The listing builds one solid part. Answer for the finished solid, in the listing's coordinates (mm). A direction names the side the tool comes from. Coordinates: 2 decimals unless noted, no trailing zeros. Order: outer loops, then holes, each group sorted by start corner. A loop starts at its lowest first (then second) coordinate and runs counter-clockwise, first axis right, second up. Notation, with made-up numbers: (18.5, 21.5) -> (53.5, 21.5) arc R14 ccw to (53.5, 27.5) -> close; hole circle Ø2 at (25.25, 50). An arc over 180 degrees is marked (long way). Return JSON: item names as keys, results as strings.
```python
from build123d import *

# Parameters (mm, degrees)
BOSS_EXTRUDE1_DEPTH     = 130
CUT_EXTRUDE3_DEPTH      = 273.019096875
CUT_EXTRUDE3_DEPTH_BACK = 273.019096875
FILLET2_SIZE            = 10
CUT_EXTRUDE4_DEPTH      = 272.254010875
CUT_EXTRUDE4_DEPTH_BACK = 272.254010875
SKETCH8_R               = 1.5
SKETCH9_W               = 24.273397223
SKETCH9_H               = 9.918939499
BOSS_EXTRUDE5_DEPTH     = 129
FILLET5_SIZE            = 5


with BuildPart() as part:
    # Sketch1 → Boss-Extrude1 (new body)
    with BuildSketch(Plane.XY):
        with BuildLine():
            Line((-213.038141425, 15.471509733), (-219.113768434, 15.471509733))
            ThreePointArc((-219.113768434, 15.471509733), (-235.448907683, -9.805845818), (-219.370745969, -35.247429766))
            Line((-219.370745969, -35.247429766), (-184.542720563, -35.247429766))
            Line((-184.542720563, -35.247429766), (-184.542720563, -25.247429766))
            Line((-184.542720563, -25.247429766), (-211.872100418, -25.247429766))
            ThreePointArc((-211.872100418, -25.247429766), (-224.566556185, -9.701816168), (-213.038141425, 6.727151008))
            Line((-213.038141425, 6.727151008), (-184.542720563, 6.727151008))
            Line((-184.542720563, 6.727151008), (-184.542720563, 15.471509733))
            Line((-184.542720563, 15.471509733), (-213.038141425, 15.471509733))
        make_face()
    extrude(amount=BOSS_EXTRUDE1_DEPTH)

    # Sketch6 → Cut-Extrude3 (cut, two sides: drawn at the far end of the back side and taken through both)
    with BuildSketch(Plane(origin=(0, -25.247429766, 0), x_dir=(1, 0, 0), z_dir=(0, 1, 0)).offset(-CUT_EXTRUDE3_DEPTH_BACK)):
        Polygon((-184.285743028, -5.850012024), (-219.113768434, -5.85), (-219.113768434, -124.15), (-184.232404978, -124.15), align=None)
    extrude(amount=CUT_EXTRUDE3_DEPTH + CUT_EXTRUDE3_DEPTH_BACK, mode=Mode.SUBTRACT)

    # loft from a face of the part (loft4)
    loft([part.faces().sort_by_distance((-198.20741049, -25.247429766, 127.075))[0], part.faces().sort_by_distance((-198.790430994, 6.727151008, 127.075))[0]])

    # loft from a face of the part (loft5)
    loft([part.faces().sort_by_distance((-198.207406817, -25.247429766, 2.925003609))[0], part.faces().sort_by_distance((-198.790427001, 6.727151008, 2.925003508))[0]])

    # Fillet2
    # a fillet whose section is not a circle: 10 mm, written as the material it takes off along each edge
    with BuildSketch(Plane(origin=(-184.542720563, 15.471509733, 99.15), x_dir=(0, -1, 0), z_dir=(0, 0, 1))) as fillet2_piece_1:
        with BuildLine():
            Bezier((FILLET2_SIZE, 0), (0, 0), (0, -FILLET2_SIZE), weights=[1, 0.353553391, 1])
            Line((0, -FILLET2_SIZE), (0, 0))
            Line((0, 0), (FILLET2_SIZE, 0))
        make_face()
    extrude(amount=55.85, mode=Mode.SUBTRACT)
    with BuildSketch(Plane(origin=(-184.542720563, -35.247429766, 99.15), x_dir=(0, 1, 0), z_dir=(0, 0, 1))) as fillet2_piece_2:
        with BuildLine():
            Bezier((FILLET2_SIZE, 0), (0, 0), (0, FILLET2_SIZE), weights=[1, 0.353553391, 1])
            Line((0, FILLET2_SIZE), (0, 0))
            Line((0, 0), (FILLET2_SIZE, 0))
        make_face()
    extrude(amount=55.85, mode=Mode.SUBTRACT)
    with BuildSketch(Plane(origin=(-184.542720563, 15.471509733, -25), x_dir=(-1, 0, 0), z_dir=(0, 0, 1))) as fillet2_piece_3:
        with BuildLine():
            Bezier((FILLET2_SIZE, 0), (0, 0), (0, FILLET2_SIZE), weights=[1, 0.353553391, 1])
            Line((0, FILLET2_SIZE), (0, 0))
            Line((0, 0), (FILLET2_SIZE, 0))
        make_face()
    extrude(amount=55.850011936, mode=Mode.SUBTRACT)
    with BuildSketch(Plane(origin=(-184.542720563, -35.247429766, -25), x_dir=(-1, 0, 0), z_dir=(0, 0, 1))) as fillet2_piece_4:
        with BuildLine():
            Bezier((FILLET2_SIZE, 0), (0, 0), (0, -FILLET2_SIZE), weights=[1, 0.353553391, 1])
            Line((0, -FILLET2_SIZE), (0, 0))
            Line((0, 0), (FILLET2_SIZE, 0))
        make_face()
    extrude(amount=55.850011936, mode=Mode.SUBTRACT)

    # Sketch8 → Cut-Extrude4 (cut, two sides: drawn at the far end of the back side and taken through both)
    with BuildSketch(Plane.XY.offset(130).offset(-CUT_EXTRUDE4_DEPTH_BACK)):
        with Locations((-198.542720563, -0.028490267)):
            Circle(SKETCH8_R)
        with Locations((-198.542720563, -20.028490267)):
            Circle(SKETCH8_R)
    extrude(amount=CUT_EXTRUDE4_DEPTH + CUT_EXTRUDE4_DEPTH_BACK, mode=Mode.SUBTRACT)

    # Sketch9 → Boss-Extrude5 (add)
    with BuildSketch(Plane.XY.offset(130)):
        with Locations((-207.234047358, -30.287960017)):
            Rectangle(SKETCH9_W, SKETCH9_H)
    extrude(amount=-BOSS_EXTRUDE5_DEPTH)

    # Fillet5
    # a fillet whose section is not a circle: 5 mm, written as the material it takes off along each edge
    with BuildSketch(Plane(origin=(-219.113768434, 3.222415949, 124.15), x_dir=(-0.7039216353317727, -0.7102776438209518, 0), z_dir=(0, 0, -1))) as fillet5_piece_1_section:
        with BuildLine():
            Bezier((1.79521773, 0), (-0.103639657, 0.102712225), (-1.454327272, 1.441313042), weights=[1, 0.23367054, 1])
            Line((-1.454327272, 1.441313042), (0, 0))
            ThreePointArc((0, 0), (0.897608865, 0.024258816), (1.79521773, 0))
        make_face()
    fillet5_piece_1 = extrude(amount=123.418868953, mode=Mode.PRIVATE)
    fillet5_piece_1 = split(fillet5_piece_1, bisect_by=Plane(origin=(-219.113727591, 3.222415949, 5.85), z_dir=(-3.452476154533893e-07, 0, 0.9999999999999404)), keep=Keep.TOP, mode=Mode.PRIVATE)
    add(fillet5_piece_1, mode=Mode.SUBTRACT)
    with BuildSketch(Plane(origin=(-195.097348746, -25.328490267, 124.15), x_dir=(-1, 0, 0), z_dir=(0, 0, -1))) as fillet5_piece_2_section:
        with BuildLine():
            Bezier((FILLET5_SIZE, 0), (0, 0), (0, -FILLET5_SIZE), weights=[1, 0.176776695, 1])
            Line((0, -FILLET5_SIZE), (0, 0))
            Line((0, 0), (FILLET5_SIZE, 0))
        make_face()
    fillet5_piece_2 = extrude(amount=130.799991708, mode=Mode.PRIVATE)
    fillet5_piece_2 = split(fillet5_piece_2, bisect_by=Plane(origin=(-195.097307903, -25.328490267, 5.850008292), z_dir=(-3.452476154533893e-07, 0, 0.9999999999999404)), keep=Keep.TOP, mode=Mode.PRIVATE)
    add(fillet5_piece_2, mode=Mode.SUBTRACT)
    with BuildSketch(Plane(origin=(-219.113768434, 15.471509733, -20.605653446), x_dir=(0, -1, 0), z_dir=(0, 0, 1))) as fillet5_piece_3_section:
        with BuildLine():
            Bezier((9.588913957, 0), (-2.904204754, 0), (6.139263069, -8.619379609), weights=[1, 0.092891751, 1])
            ThreePointArc((6.139263069, -8.619379609), (2.657898383, -4.602951994), (0, 0))
            Line((0, 0), (9.588913957, 0))
        make_face()
    fillet5_piece_3 = extrude(amount=144.755653446, mode=Mode.PRIVATE)
    fillet5_piece_3 = split(fillet5_piece_3, bisect_by=Plane(origin=(-219.113777568, 15.471509733, 5.85), z_dir=(-3.452476154533893e-07, 0, 0.9999999999999404)), keep=Keep.TOP, mode=Mode.PRIVATE)
    add(fillet5_piece_3, mode=Mode.SUBTRACT)


solid = part.part
```
Item 1: Determine the mould class of faces 4 (the flat face through (-210, -25.328, 66)), 5 (the flat face through (-212.463, -9.036, 127.116)), 6 (the flat face through (-210, -10, 0)) for opening direction Z: pulls with the +Z half, pulls with the -Z half, needs draft (parallel to the pull), parting line crosses it, or undercut.
Answer list:
{"face 4": "undercut", "face 5": "needs draft", "face 6": "pulls with the -Z half"}
Item 2: Flat-ended cylindrical pins translate along their axes: pin 1 (1 mm diameter, centred on y = -17.5, z = 38.5, fed in from +X); pin 2 (10 mm diameter, centred on x = -206.5, z = 101, fed in from +Y); pin 3 (4.5 mm diameter, centred on y = -24, z = 36.5, fed in from +X); pin 4 (2.5 mm diameter, centred on x = -198.54, y = -0.03, fed in from -Z). Find the tip coordinate at first contact, or state that the pin passes through.
Answer list:
{"pin 1": "x = -221.99", "pin 2": "y = -25.33", "pin 3": "x = -198.55", "pin 4": "through"}
Item 3: The part is cut by section B-B on y = -16. Count the separate pieces of the cut face and the enclosed holes in it, plus the area to 3 significant figures.
Answer list:
{"separate pieces": "3", "enclosed holes": "0", "area": "1,850 mm2"}
Item 4: Find the intervals of material crossed by probe 1 along Z at (x, y) = (-206.5, 2); probe 2 along Y at (x, z) = (-211, 48.5), in increasing order.
Answer list:
{"probe 1": "0 to 5.85, 124.15 to 130", "probe 2": "-35.25 to -25.33"}
Item 5: Which of the six approach directions +Z, -Z, +X, -X, +Y, -Y give full straight-line access (tool end or side, diameter ignored) to faces 1 (the flat face through (-219.114, -23, 64)), 2 (the cylindrical face through (-197.157, -20.603, 2.884)), 3 (the flat face through (-195.097, -33, 66))?
Answer list:
{"face 1": "+X, +Y", "face 2": "+Z, -Z", "face 3": "+X, +Y, -Y"}
Item 6: The part is cut by section A-A on x = -215.5. Determine the outline of the cut face in (y, z).
Answer list:
{"outline": "(-35.25, 0) -> (-23.91, 0) -> (-23.91, 5.85) -> (-25.33, 5.85) -> (-25.33, 124.15) -> (-23.91, 124.15) -> (-23.91, 130) -> (-35.25, 130) -> close; (5.71, 0) -> (15.47, 0) -> (15.47, 5.85) -> (5.71, 5.85) -> close; (5.71, 124.15) -> (15.47, 124.15) -> (15.47, 130) -> (5.71, 130) -> close"}
